The model under review builds one solid part; all positions refer to its coordinate system, in mm. A direction names the side the tool comes from. Round coordinates to 2 decimals unless told otherwise and drop trailing zeros. Loops run counter-clockwise (first coordinate to the right, second up) from the corner with the lowest first, then second, coordinate; pieces in that order, holes last. Notation, with made-up numbers: (81.5, -29) -> (105.5, -29) arc R8 ccw to (105.5, -18) -> close; hole circle Ø1 at (-13, 45.25). An arc over 180 degrees is marked (long way). Use a Markdown table: item, result. Add a question column.
1) Consider section A-A on z = 0. Give the boundary of the cut face in (x, y) (3 decimals).
2) Mouldability with a two-part tool opening along Z and no side actions: class faces 1 (the flat face through (25, 20, -25)), 2 (the flat face through (-45, 20, 0)), 3 (the cylindrical face through (-0.69, 20.28, 3.1)) as released by +Z, released by -Z, zero draft, split by the parting line, or undercut.
3) For faces 4 (the cylindrical face through (15.46, 23, -22.46)), 5 (the flat face through (45, 20, 0)), list the 3-axis set-ups (+Z, -Z, +X, -X, +Y, -Y) from which the entire face can be reached by the end or side of a thin tool; tool diameter is ignored.
4) Insertion check: pin 1 (12 mm diameter, centred on x = 7, y = 30.5, fed in from -Z). The pin has a flat end and moves straight along its axis. Give the tip position at first contact, or say it passes through.
5) Consider section C-C on y = 8. Give the boundary of the cut face in (x, z) (3 decimals).
6) Consider section D-D on x = 25. Give the boundary of the cut face in (y, z).
7) Wall thickness on probe 1 along Z at (x, y) = (0, 16) (3 decimals); probe 2 along X at (y, z) = (27, 0) (3 decimals); probe 3 along Z at (x, y) = (-29, 29.5): over which ranges is each line inside the solid? List them lowest first.
8) Consider section B-B on x = 0. Give the boundary of the cut face in (y, z) (3 decimals).
from build123d import *

# Parameters (mm, degrees)
SKETCH1_W           = 90
SKETCH1_H           = 40
BOSS_EXTRUDE1_DEPTH = 40
SKETCH2_R           = 10
BOSS_EXTRUDE2_DEPTH = 5
SKETCH3_R           = 3.175
CUT_EXTRUDE1_DEPTH  = 41


with BuildPart() as part:
    # Sketch1 → Boss-Extrude1 (new body)
    with BuildSketch(Plane(origin=(0, 0, 0), x_dir=(1, 0, 0), z_dir=(0, 1, 0))):
        Rectangle(SKETCH1_W, SKETCH1_H)
    extrude(amount=BOSS_EXTRUDE1_DEPTH)

    # Sketch2 → Boss-Extrude2 (add)
    with BuildSketch(Plane(origin=(0, 0, -20), x_dir=(-1, 0, 0), z_dir=(0, 0, -1))):
        with Locations((-25, 20)):
            Circle(SKETCH2_R)
    extrude(amount=BOSS_EXTRUDE2_DEPTH)

    # Sketch3 → Cut-Extrude1 (cut, through all)
    with BuildSketch(Plane(origin=(0, 40, 0), x_dir=(1, 0, 0), z_dir=(0, 1, 0))):
        Circle(SKETCH3_R)
    extrude(amount=-CUT_EXTRUDE1_DEPTH, mode=Mode.SUBTRACT)


solid = part.part
Result set:
| question | item | result |
|---|---|---|
| 1 | outline | (-45, 0) -> (-3.175, 0) -> (-3.175, 40) -> (-45, 40) -> close; (3.175, 0) -> (45, 0) -> (45, 40) -> (3.175, 40) -> close |
| 2 | face 1 | released by -Z |
| 2 | face 2 | zero draft |
| 2 | face 3 | undercut |
| 3 | face 4 | -Z |
| 3 | face 5 | +Z, -Z, +X, +Y, -Y |
| 4 | pin 1 | z = -20 |
| 5 | outline | (-45, -20) -> (45, -20) -> (45, 20) -> (-45, 20) -> close; hole circle Ø6.35 at (0, 0) |
| 6 | outline | (0, -20) -> (10, -20) -> (10, -25) -> (30, -25) -> (30, -20) -> (40, -20) -> (40, 20) -> (0, 20) -> close |
| 7 | probe 1 | -20 to -3.175, 3.175 to 20 |
| 7 | probe 2 | -45 to -3.175, 3.175 to 45 |
| 7 | probe 3 | -20 to 20 |
| 8 | outline | (0, -20) -> (40, -20) -> (40, -3.175) -> (0, -3.175) -> close; (0, 3.175) -> (40, 3.175) -> (40, 20) -> (0, 20) -> close |
